Verification items for the finished model (mm, model axes). A direction names the side the tool comes from. Coordinates: 2 decimals unless noted, no trailing zeros. Write each loop counter-clockwise with the first axis right and the second up, starting at its lowest first coordinate (ties: lowest second). Pieces come first, ordered by that corner, then holes. Notation, with made-up numbers: (40.5, 79.5) -> (54.5, 79.5) arc R28 cw to (54.5, 104.5) -> close; hole circle Ø9 at (-9, 64.5). An arc over 180 degrees is marked (long way). Write item = value, one per line. Start each with the question number.
(1) Gauge pin test, flat ends, axial feed: pin 1 Ø0.8 at (x, z) = (-50, 4.5) entering from +Y; pin 2 Ø1.9 at (y, z) = (-42, 2) entering from -X; pin 3 Ø1.3 at (x, z) = (-50.5, 5) entering from -Y. Record the tip position at first contact, or that the pin passes through.
(2) Section check A-A (x = -43). Record the cut outline in (y, z).
(3) Mould release check, pull along Y, two halves, no side actions. Record for faces 1 (the face through (-42.892, -46.307, 3.131)), 2 (the face through (-42, -25, 0)), 3 (the face through (-50, -6.244, 3)): released by +Y, released by -Y, zero draft, split by the parting line, or undercut.
(4) Material ranges on probe 1 along Y at (x, z) = (-35, 3.75); probe 2 along X at (y, z) = (-43.5, 5.25); probe 3 along X at (y, z) = (-44.5, 3.5), recorded low to high. Write a range as [from, to].
(5) Section check D-D (x = -48.25). Record the cut outline in (y, z), plus the area to 3 significant figures.
(6) Section check C-C (y = -36). Record the cut outline in (x, z).
(7) Section check B-B (z = 0.5). State how many separate pieces and enclosed holes the cut face has, plus the area to 3 significant figures.
(8) Set-up check for faces 4 (the face through (-50, -30.311, 3)), 5 (the face through (-39, -48.762, 3)): record each of +Z, -Z, +X, -X, +Y, -Y from which the full face is reachable in a straight line by a thin tool's end or side.
```python
from build123d import *

# Parameters (mm, degrees)
SKETCH1_R           = 1.1684
SKETCH1_R_2         = 0.889
BOSS_EXTRUDE1_DEPTH = 6.35


with BuildPart() as part:
    # Sketch1 → Boss-Extrude1 (new body)
    with BuildSketch(Plane.XY):
        with BuildLine():
            Line((-31.453240404, -3.582490692), (-31.453240404, -46.222490692))
            ThreePointArc((-31.453240404, -46.222490692), (-32.197189179, -48.018541916), (-33.993240404, -48.762490692))
            Line((-33.993240404, -48.762490692), (-44.383240404, -48.762490692))
            ThreePointArc((-44.383240404, -48.762490692), (-46.179291628, -48.018541916), (-46.923240404, -46.222490692))
            Line((-46.923240404, -46.222490692), (-46.923240404, -32.850740692))
            ThreePointArc((-46.923240404, -32.850740692), (-47.667189179, -31.054689467), (-49.463240404, -30.310740692))
            Line((-49.463240404, -30.310740692), (-51.065740404, -30.310740692))
            ThreePointArc((-51.065740404, -30.310740692), (-52.861791628, -29.566791916), (-53.605740404, -27.770740692))
            Line((-53.605740404, -27.770740692), (-53.605740404, -8.784240692))
            ThreePointArc((-53.605740404, -8.784240692), (-52.861791628, -6.988189467), (-51.065740404, -6.244240692))
            Line((-51.065740404, -6.244240692), (-49.463240404, -6.244240692))
            ThreePointArc((-49.463240404, -6.244240692), (-47.667189179, -5.500291916), (-46.923240404, -3.704240692))
            Line((-46.923240404, -3.704240692), (-46.923240404, -3.582490692))
            ThreePointArc((-46.923240404, -3.582490692), (-46.179291628, -1.786439467), (-44.383240404, -1.042490692))
            Line((-44.383240404, -1.042490692), (-33.993240404, -1.042490692))
            ThreePointArc((-33.993240404, -1.042490692), (-32.197189179, -1.786439467), (-31.453240404, -3.582490692))
        make_face()
        with Locations((-43.430740404, -4.534990692)):
            Circle(SKETCH1_R, mode=Mode.SUBTRACT)
        with Locations((-34.945740404, -4.534990692)):
            Circle(SKETCH1_R, mode=Mode.SUBTRACT)
        with Locations((-43.430740404, -45.269990692)):
            Circle(SKETCH1_R, mode=Mode.SUBTRACT)
        with Locations((-34.945740404, -45.269990692)):
            Circle(SKETCH1_R, mode=Mode.SUBTRACT)
        with Locations((-50.113240404, -9.736740692)):
            Circle(SKETCH1_R_2, mode=Mode.SUBTRACT)
        with Locations((-50.113240404, -26.818240692)):
            Circle(SKETCH1_R_2, mode=Mode.SUBTRACT)
    extrude(amount=BOSS_EXTRUDE1_DEPTH)


solid = part.part
```
Response:
q1.pin_1 = -6.24
q1.pin_2 = -46.92
q1.pin_3 = -30.31
q2.outline = (-48.76, 0) -> (-46.36, 0) -> (-46.36, 6.35) -> (-48.76, 6.35) -> close; (-44.18, 0) -> (-5.62, 0) -> (-5.62, 6.35) -> (-44.18, 6.35) -> close; (-3.45, 0) -> (-1.04, 0) -> (-1.04, 6.35) -> (-3.45, 6.35) -> close
q3.face_1 = undercut
q3.face_2 = zero draft
q3.face_3 = released by +Y
q4.probe_1 = [-48.76, -46.44], [-44.1, -5.7], [-3.37, -1.04]
q4.probe_2 = [-46.92, -31.45]
q4.probe_3 = [-46.92, -44.31], [-42.55, -35.82], [-34.07, -31.45]
q5.outline = (-30.62, 0) -> (-5.94, 0) -> (-5.94, 6.35) -> (-30.62, 6.35) -> close
q5.area = 157 mm2
q6.outline = (-46.92, 0) -> (-31.45, 0) -> (-31.45, 6.35) -> (-46.92, 6.35) -> close
q7.separate_pieces = 1
q7.enclosed_holes = 6
q7.area = 871 mm2
q8.face_4 = +Z, -Z, -X, -Y
q8.face_5 = +Z, -Z, +X, -X, -Y
